For this review, use the dimensioned drawing (mm, ordinates from the lowest corner) and the shaded views. Coordinates: 2 decimals unless noted, no trailing zeros. Loops run counter-clockwise (first coordinate to the right, second up) from the corner with the lowest first, then second, coordinate; pieces in that order, holes last. Notation, with made-up numbers: (11.25, -29) - (45.25, -29) arc R22 cw to (45.25, 6) - close; hole circle Ø9 at (-16, -35.5). An arc over 180 degrees is marked (long way). Answer in a Markdown table with one row per item. Add a question column.
(1) To check wall thickness, follow L1, parallel to X at y = 103.5, z = 1.8; L2, parallel to X at y = 113.5, z = 2.15; L3, parallel to Y at x = 8.25, z = 1.75. State the ranges of each line that lie inside material, in increasing order. Write a range as [from, to].
(2) We need section B-B, the plane y = 31.5. Write out the cut boundary in (x, z), plus the area to 3 significant figures.
(3) We need section A-A, the plane z = 2.35. Give the number of separate pieces and of enclosed holes in the cut face, plus the area to 3 significant figures.
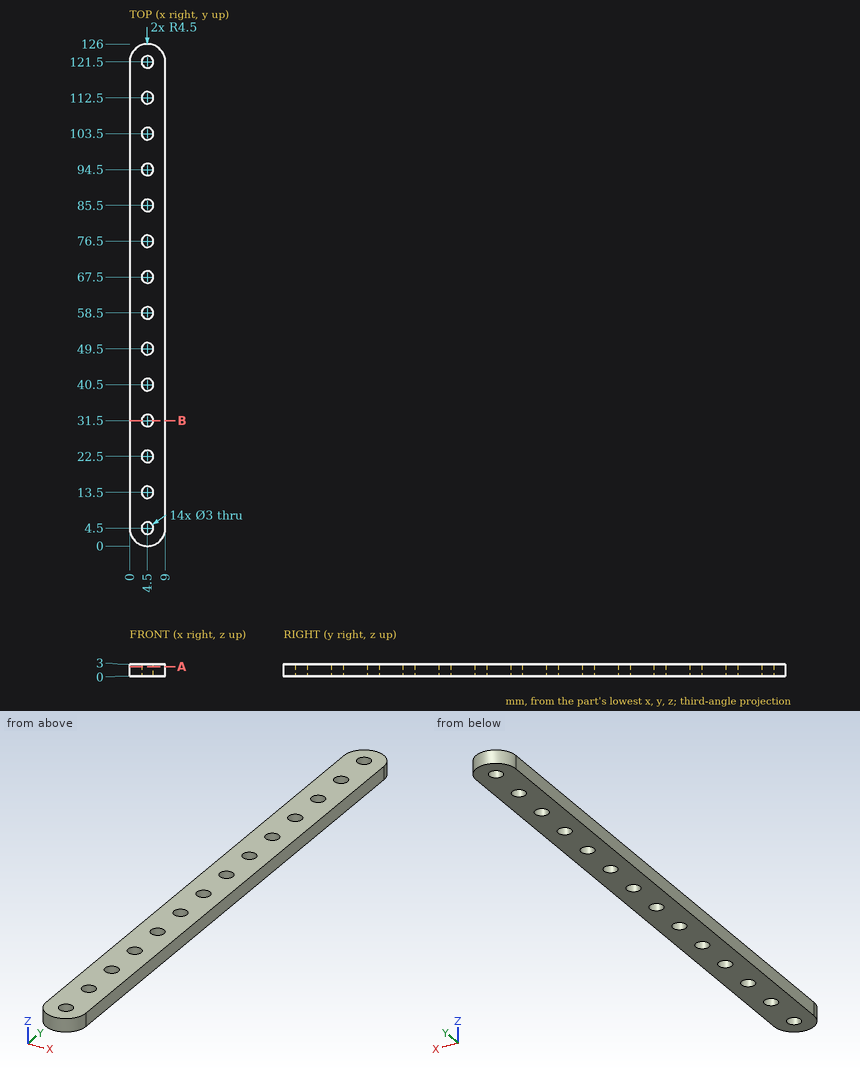
Responses:
| question | item | result |
|---|---|---|
| 1 | L1 | x = [0, 3], [6, 9] |
| 1 | L2 | x = [0, 3.38], [5.62, 9] |
| 1 | L3 | y = [2.01, 123.99] |
| 2 | outline | (0, 0) - (3, 0) - (3, 3) - (0, 3) - close; (6, 0) - (9, 0) - (9, 3) - (6, 3) - close |
| 2 | area | 18.0 mm2 |
| 3 | separate pieces | 1 |
| 3 | enclosed holes | 14 |
| 3 | area | 1,020 mm2 |
